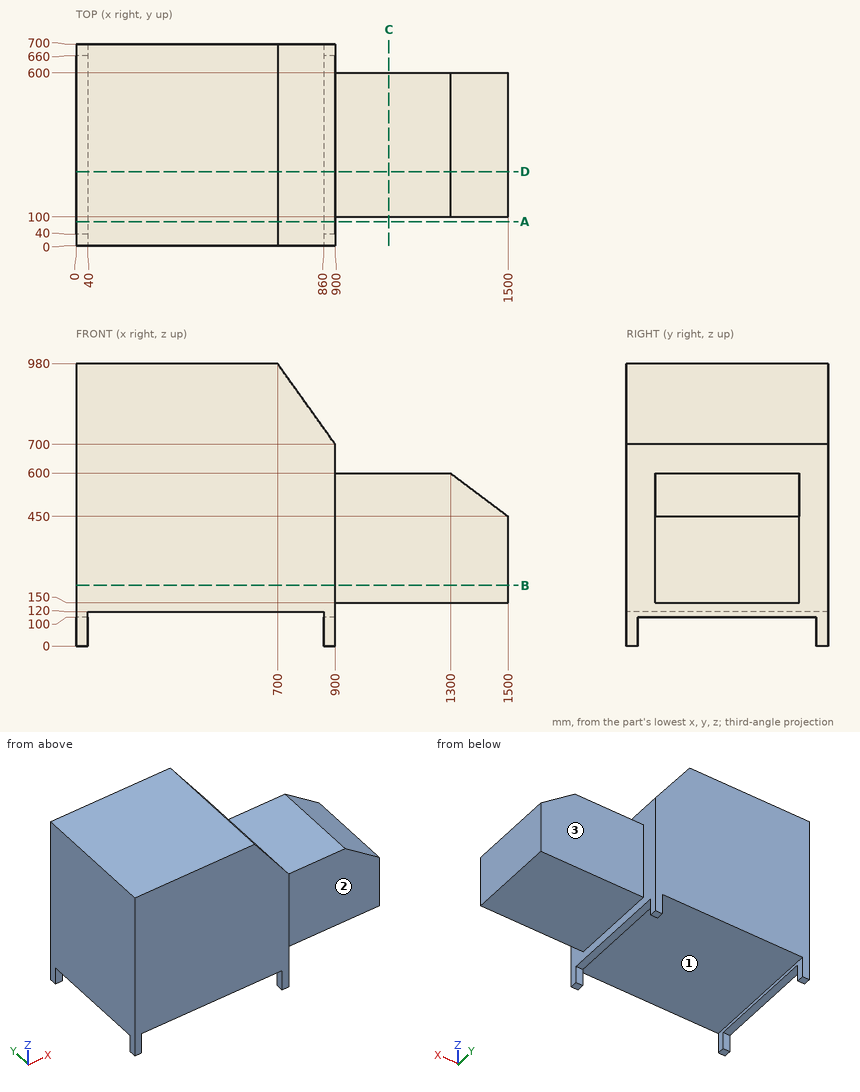
Part print with two shaded views. Sizes in mm from the minimum x, y, z corner. A direction names the side the tool comes from. Coordinates: 2 decimals unless noted, no trailing zeros. Write each loop counter-clockwise with the first axis right and the second up, starting at its lowest first coordinate (ties: lowest second). Pieces come first, ordered by that corner, then holes. Notation, with made-up numbers: (-2, -9) -> (48, -9) arc R30 ccw to (48, 15) -> close; hole circle Ø7 at (9.5, -16.5). An arc over 180 degrees is marked (long way). Return JSON: item names as keys, results as strings. Group by question number.
Q1. Cut at A-A, the plane y = 83.5. Give the cut face in (x, z), then the cut area to 3 significant figures.
Q2. Cut at D-D, the plane y = 257.5. Give the cut face in (x, z).
Q3. Drill centre lines: line 1 (Z direction, x = 158, y = 96); line 2 (X direction, y = 178.5, z = 678.5); line 3 (Z direction, x = 927.5, y = 451.5). Where is each one in solid material? Low to high.
Q4. Cut at C-C, the plane x = 1085.5. Give the cut face in (y, z).
Q5. Cut at B-B, the plane z = 210.5. Give the cut face in (x, y), then the cut area to 3 significant figures.
Q6. Flat gauge pins, fed straight in: pin 1 (12 mm diameter, centred on y = 285.5, z = 137.5, fed in from +X); pin 2 (3 mm diameter, centred on x = 947.5, y = 501, fed in from +Z); pin 3 (1 mm diameter, centred on y = 481.5, z = 527.5, fed in from +X). Where does each tip first touch, or does it go through?
Q7. Which spindle directions (+Z, -Z, +X, -X, +Y, -Y) get a long thin tool onto all of the face, cutting with end or side? Do the marked faces 1, 2 and 3. Say none if no direction does.
Returned:
{
 "1": {"outline": "(0, 100) -> (40, 100) -> (40, 120) -> (860, 120) -> (860, 100) -> (900, 100) -> (900, 700) -> (700, 980) -> (0, 980) -> close", "area": "748,000 mm2"},
 "2": {"outline": "(0, 100) -> (40, 100) -> (40, 120) -> (860, 120) -> (860, 100) -> (900, 100) -> (900, 150) -> (1500, 150) -> (1500, 450) -> (1300, 600) -> (900, 600) -> (900, 700) -> (700, 980) -> (0, 980) -> close"},
 "3": {"line 1": "z = 120 to 980", "line 2": "x = 0 to 900", "line 3": "z = 150 to 600"},
 "4": {"outline": "(100, 150) -> (600, 150) -> (600, 600) -> (100, 600) -> close"},
 "5": {"outline": "(0, 0) -> (900, 0) -> (900, 100) -> (1500, 100) -> (1500, 600) -> (900, 600) -> (900, 700) -> (0, 700) -> close", "area": "930,000 mm2"},
 "6": {"pin 1": "stops at x = 900", "pin 2": "stops at z = 600", "pin 3": "stops at x = 1397.33"},
 "7": {"face 1": "-Z, +Y, -Y", "face 2": "+Z, -Z, +X, -Y", "face 3": "+Z, -Z, +X, +Y"}
}
